```python
from build123d import *

# Parameters (mm, degrees)
BOSS_EXTRUDE2_DEPTH = 10
SKETCH3_W           = 4.3
SKETCH3_H           = 5
CUT_EXTRUDE3_DEPTH  = 4.3
SKETCH5_R           = 1.5
SKETCH5_W           = 4
SKETCH5_H           = 0.25
CUT_EXTRUDE4_DEPTH  = 5.3


with BuildPart() as part:
    # Sketch2 → Boss-Extrude2 (new body)
    with BuildSketch(Plane.XY):
        Polygon((-3.311102547, 0), (3.311102547, 0), (3.311102547, 6.2), (2.933626588, 10.202238361), (-1.766373412, 10.202238361), (-3.311102547, 6.2), align=None)
    extrude(amount=BOSS_EXTRUDE2_DEPTH)

    # Sketch3 → Cut-Extrude3 (cut)
    with BuildSketch(Plane(origin=(0, 0, 0), x_dir=(0, 0, -1), z_dir=(1, 0, 0))):
        with Locations((-2.5, 3.1)):
            Rectangle(SKETCH3_W, SKETCH3_H)
        with Locations((-7.5, 3.1)):
            Rectangle(SKETCH3_W, SKETCH3_H)
    extrude(amount=CUT_EXTRUDE3_DEPTH, mode=Mode.SUBTRACT)

    # Sketch5 → Cut-Extrude4 (cut)
    with BuildSketch(Plane(origin=(0, 10.202238361, 0), x_dir=(1, 0, 0), z_dir=(0, 1, 0))):
        with Locations((0.583626588, -7.15)):
            Circle(SKETCH5_R)
        with Locations((0.583626588, -5.125)):
            Rectangle(SKETCH5_W, SKETCH5_H)
        with Locations((0.583626588, -4.875)):
            Rectangle(SKETCH5_W, SKETCH5_H)
        with Locations((0.583626588, -2.85)):
            Circle(SKETCH5_R)
    extrude(amount=-CUT_EXTRUDE4_DEPTH, mode=Mode.SUBTRACT)


solid = part.part
```
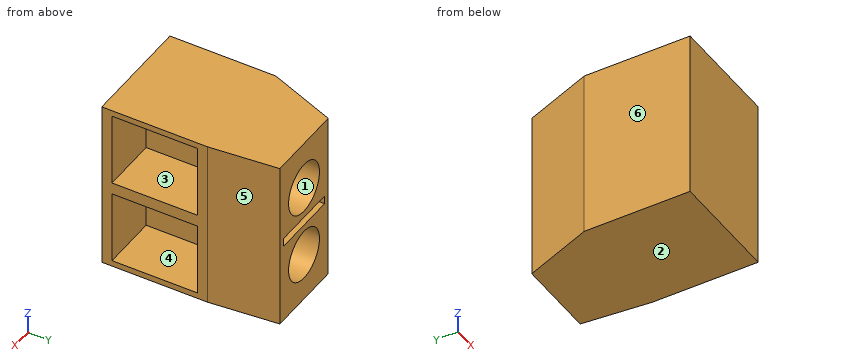
Design review of the part built by this model. Coordinates are the model's own, in mm. Face numbers are marked on the shaded views. A direction names the side the tool comes from. Coordinates: 2 decimals unless noted, no trailing zeros. Order: outer loops, then holes, each group sorted by start corner. A loop starts at its lowest first (then second) coordinate and runs counter-clockwise, first axis right, second up. Notation, with made-up numbers: (55, -14.75) -> (62, -14.75) arc R5 cw to (62, -8.75) -> close; hole circle Ø4 at (43.25, 66.25). An arc over 180 degrees is marked (long way). One line per item, written item: value. Start each with the question number.
Q1. For probe 1 along Z at (x, y) = (3, 2); probe 2 along Y at (x, z) = (1.5, 1.5); probe 3 along Z at (x, y) = (0.25, 7.5), list the stretches that pass through material, from the lowest coordinate up.
Q2. Take a section at B-B, the plane z = 2.5. State the section outline as (x, y) points, then the cut area to 3 significant figures.
Q3. Tool access review of the marked faces 1, 2 and 3: name each direction out of +Z, -Z, +X, -X, +Y, -Y from which nothing blocks a thin tool from reaching the whole face with its end or side.
Q4. Take a section at D-D, the plane y = 1.25. State the section outline as (x, z) points, then the cut area to 3 significant figures.
Q5. Take a section at C-C, the plane x = 2.25. State the section outline as (y, z) points, then the cut area to 3 significant figures.
Q6. Mouldability with a two-part tool opening along Y and no side actions: class the marked faces 4, 5 and 6 as pulls with the +Y half, pulls with the -Y half, needs draft (parallel to the pull), parting line crosses it, or undercut.
Q7. Take a section at A-A, the plane y = 6. State the section outline as (x, z) points, then the cut area to 3 significant figures.
Q8. Insertion check: pin 1 Ø3 at (x, y) = (1, 7) entering from -Z; pin 2 Ø2.5 at (x, z) = (0.58, 2.85) entering from +Y. Each pin has a flat end and moves straight along its axis. Give the tip position at first contact, or say it passes through.
Values follow:
1. probe 1: z = 0 to 0.35, 4.65 to 5.35, 9.65 to 10
1. probe 2: y = 0 to 0.6, 5.6 to 10.2
1. probe 3: z = 0 to 1.39, 4.31 to 4.75, 5.25 to 5.69, 8.61 to 10
2. outline: (-3.31, 0) -> (3.31, 0) -> (3.31, 0.6) -> (0, 0.6) -> (0, 4.9) -> (-0.87, 4.9) -> (-0.87, 10.2) -> (-1.77, 10.2) -> (-3.31, 6.2) -> close; (2.04, 5.6) -> (3.31, 5.6) -> (3.31, 6.2) -> (2.93, 10.2) -> (2.04, 10.2) -> close
2. area: 33.1 mm2
3. face 1: +Y
3. face 2: -Z, +X, -X, +Y, -Y
3. face 3: +X
4. outline: (-3.31, 0) -> (3.31, 0) -> (3.31, 0.35) -> (0, 0.35) -> (0, 4.65) -> (3.31, 4.65) -> (3.31, 5.35) -> (0, 5.35) -> (0, 9.65) -> (3.31, 9.65) -> (3.31, 10) -> (-3.31, 10) -> close
4. area: 37.7 mm2
5. outline: (0, 0) -> (10.2, 0) -> (10.2, 4.75) -> (4.9, 4.75) -> (4.9, 5.25) -> (10.2, 5.25) -> (10.2, 10) -> (0, 10) -> close; hole (0.6, 0.35) -> (5.6, 0.35) -> (5.6, 4.65) -> (0.6, 4.65) -> close; hole (0.6, 5.35) -> (5.6, 5.35) -> (5.6, 9.65) -> (0.6, 9.65) -> close
5. area: 56.4 mm2
6. face 4: undercut
6. face 5: pulls with the +Y half
6. face 6: needs draft
7. outline: (-3.31, 0) -> (3.31, 0) -> (3.31, 10) -> (-3.31, 10) -> close; hole (-1.42, 4.75) -> (2.58, 4.75) -> (2.58, 5.25) -> (-1.42, 5.25) -> close; hole circle Ø3 at (0.58, 2.85); hole circle Ø3 at (0.58, 7.15)
7. area: 50.1 mm2
8. pin 1: stops at z = 0
8. pin 2: stops at y = 4.9
